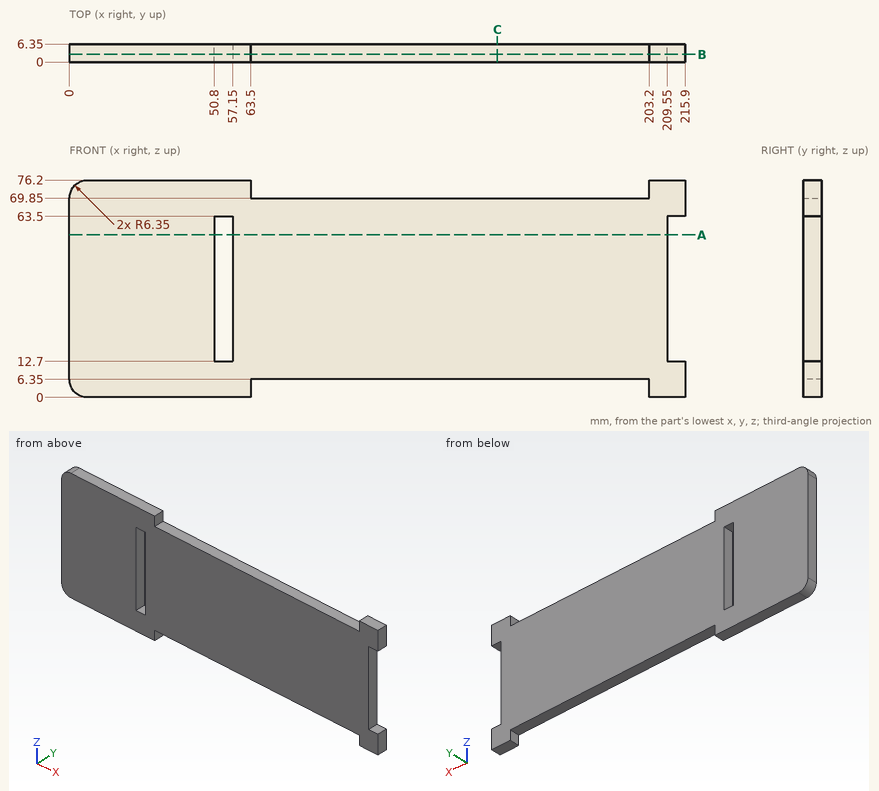
Geometry check sheet. Reference: drawing and pictorial views, mm from the part's lowest x, y, z. Round coordinates to 2 decimals unless told otherwise and drop trailing zeros. Loops run counter-clockwise (first coordinate to the right, second up) from the corner with the lowest first, then second, coordinate; pieces in that order, holes last. Notation, with made-up numbers: M 19,-36 L 38,-36 A7 cw 38,-32 Z; hole C 13.5,-13.75 d2. An arc over 180 degrees is marked long. One line per item, written item: value.
(1) Thickness scan on line 1 (X direction, y = 4.5, z = 14.5); line 2 (Z direction, x = 88, y = 4.25); line 3 (X direction, y = 6, z = 4.5). Record the ranges inside material, lowest first.
Computed values:
line 1: x = 0 to 50.8, 57.15 to 209.55
line 2: z = 6.35 to 69.85
line 3: x = 0.28 to 63.5, 203.2 to 215.9
(2) Sectioned sample at A-A, the plane z = 57. Record the cut outline in (x, y).
Computed values:
outline: M 0,0 L 50.8,0 L 50.8,6.35 L 0,6.35 Z; M 57.15,0 L 209.55,0 L 209.55,6.35 L 57.15,6.35 Z
(3) Depth check by flat-ended pin: pin 1 Ø1 at (x, y) = (136, 3) entering from +Z; pin 2 Ø1.5 at (x, y) = (181.5, 2.5) entering from -Z; pin 3 Ø1 at (y, z) = (1.5, 26.5) entering from +X. Enter the tip coordinate at first touch or a pass-through.
Computed values:
pin 1: stops at z = 69.85
pin 2: stops at z = 6.35
pin 3: stops at x = 209.55
(4) Sectioned sample at C-C, the plane x = 150. Record the cut outline in (y, z).
Computed values:
outline: M 0,6.35 L 6.35,6.35 L 6.35,69.85 L 0,69.85 Z
(5) Sectioned sample at B-B, the plane y = 2.75. Record the cut outline in (x, z).
Computed values:
outline: M 0,6.35 A6.35 ccw 6.35,0 L 63.5,0 L 63.5,6.35 L 203.2,6.35 L 203.2,0 L 215.9,0 L 215.9,12.7 L 209.55,12.7 L 209.55,63.5 L 215.9,63.5 L 215.9,76.2 L 203.2,76.2 L 203.2,69.85 L 63.5,69.85 L 63.5,76.2 L 6.35,76.2 A6.35 ccw 0,69.85 Z; hole M 50.8,12.7 L 57.15,12.7 L 57.15,63.5 L 50.8,63.5 Z
